```python
from build123d import *

# Parameters (mm, degrees)
BOSS_EXTRUDE2_DEPTH    = 3
FILLET1_R              = 1
LPATTERN1_COUNT        = 3
LPATTERN1_PITCH        = 37.5
FILLET1_OF_LPATTERN1_R = 1


with BuildPart() as part:
    # Sketch2 → Boss-Extrude2 (new body)
    with BuildSketch(Plane(origin=(0, 0, 0), x_dir=(0, 0, -1), z_dir=(1, 0, 0))):
        Polygon((-4, 102), (-4, 108), (-11, 108), (-12, 118), (-18.75, 118), (-18.75, -103), (18.75, -103), (18.75, 118), (12, 118), (11, 108), (4, 108), (4, 102), align=None)
    boss_extrude2 = extrude(amount=BOSS_EXTRUDE2_DEPTH)

    # Fillet1
    fillet1_edges = [part.edges().sort_by_distance(p)[0] for p in [
        (1.5, 108, -4),
        (1.5, 118, -12),
        (1.5, 118, 12),
        (1.5, 108, 4),
        (1.5, 102, 4),
        (1.5, 102, -4),
    ]]
    fillet(fillet1_edges, radius=FILLET1_R)

    # LPattern1: Boss-Extrude2 ×3
    with Locations(*[(0, 0, i * LPATTERN1_PITCH) for i in range(1, LPATTERN1_COUNT)]):
        add(boss_extrude2)

    # Fillet1 of LPattern1
    fillet1_of_lpattern1_edges = [part.edges().sort_by_distance(p)[0] for p in [
        (1.5, 108, 33.5),
        (1.5, 118, 25.5),
        (1.5, 118, 49.5),
        (1.5, 108, 41.5),
        (1.5, 102, 41.5),
        (1.5, 102, 33.5),
        (1.5, 108, 71),
        (1.5, 118, 63),
        (1.5, 118, 87),
        (1.5, 108, 79),
        (1.5, 102, 79),
        (1.5, 102, 71),
    ]]
    fillet(fillet1_of_lpattern1_edges, radius=FILLET1_OF_LPATTERN1_R)


solid = part.part
```
The model under review builds one solid part; all positions refer to its coordinate system, in mm. Give positions to 0.01 mm unless a question says otherwise; leave off trailing zeros. Write each loop counter-clockwise with the first axis right and the second up, starting at its lowest first coordinate (ties: lowest second). Pieces come first, ordered by that corner, then holes. Notation, with made-up numbers: (57, 44) -> (104, 44) arc R9 ccw to (104, 50) -> close; hole circle Ø11 at (20.5, 85). An arc over 180 degrees is marked (long way). Answer in a Markdown table with one row per item.
1) Add section A-A on z = 74. State the section outline as (x, y) points.
Worked answers:
| item | result |
|---|---|
| outline | (0, -103) -> (3, -103) -> (3, 102) -> (0, 102) -> close |
2) For L1, parallel to Y at x = 0.85, z = 39.5; L2, parallel to Y at x = 1.45, z = -10, list the stretches that pass through material, from the lowest coordinate up. Write a range as [from, to].
Worked answers:
| item | result |
|---|---|
| L1 | [-103, 102] |
| L2 | [-103, 108] |
3) Clearance check with flat-ended pins moving along their axes: P1, Ø0.9, axis at x = 1, z = 38, coming from the +Y side; P2, Ø0.9, axis at x = 1.5, z = 29.5, coming from the +Y side. State where each tip first meets the part, or that it passes through.
Worked answers:
| item | result |
|---|---|
| P1 | y = 102 |
| P2 | y = 108 |
